Source: CAD feature listing. Evaluate the final solid. Frame: model axes, mm. A direction names the side the tool comes from. Round coordinates to 2 decimals unless told otherwise and drop trailing zeros. Order: outer loops, then holes, each group sorted by start corner. A loop starts at its lowest first (then second) coordinate and runs counter-clockwise, first axis right, second up. Notation, with made-up numbers: M -18,9.25 L 32,9.25 A24 ccw 32,44.25 Z; hole C -13,18 d11. An arc over 180 degrees is marked long. Answer as CSV lines item,"result". Start each with the question number.
Item 1: Line query: line 1 (Z direction, x = 13, y = 28); line 2 (Z direction, x = 4, y = 34); line 3 (Z direction, x = 3.5, y = 13). Output: solid intervals per line, ascending. Write a range as [from, to].
Item 2: Section query B-B on x = 11.6. Return the cut outline in (y, z), plus the area to 3 significant figures.
Item 3: Pull-direction query (X, two-part tool) for faces 5 (the face through (12, 0, 15)), 6 (the face through (11.65, 4.33, -15.21)), 7 (the face through (-12.747, 33.699, -0.28)); classes: +X half, -X half, draft (parallel to the pull), parting line (faces both ways), or undercut.
Item 4: First-contact query: P1, Ø0.6, axis at y = 0.5, z = -14.5, coming from the +X side; P2, Ø3, axis at x = 3, z = -16, coming from the +Y side; P3, Ø1.6, axis at y = 1, z = -14, coming from the -X side. Flat tips, straight axial feed; report the tip coordinate or a pass-through.
Item 5: Section query A-A on y = 26.5. Return the cut outline in (x, z), plus the area to 3 significant figures.
Item 6: Set-up query: faces 1 (the face through (35.947, 33.699, 0.28)), 2 (the face through (12, 38, -2.55)), 3 (the face through (-10.747, 16.146, -0.236)), 4 (the face through (11.8, 45.7, 7.4)). Return all of +Z, -Z, +X, -X, +Y, -Y with unobstructed straight access to the full face (end or side cutting, diameter ignored); none if empty.
from build123d import *

# Parameters (mm, degrees)
BOSS_EXTRUDE1_DEPTH     = 53.5
BOSS_EXTRUDE2_START     = 32.75
BOSS_EXTRUDE2_DEPTH     = 10
BOSS_EXTRUDE3_DEPTH     = 2
FILLET1_R               = 10.75
FILLET2_R               = 14
FILLET3_R               = 1
CUT_EXTRUDE4_DEPTH      = 79.076260797
CUT_EXTRUDE5_DEPTH      = 61.840180017
CUT_EXTRUDE5_DEPTH_BACK = 61.840180017


# Some blends are built 0.0001 mm under size
with BuildPart() as part:
    # Sketch2 → Boss-Extrude1 (new body)
    with BuildSketch(Plane(origin=(0, 0, 0), x_dir=(1, 0, 0), z_dir=(0, 1, 0))):
        with BuildLine():
            Line((0, -12.75), (23.2, -12.75))
            ThreePointArc((23.2, -12.75), (35.95, 0), (23.2, 12.75))
            Line((23.2, 12.75), (0, 12.75))
            ThreePointArc((0, 12.75), (-12.75, 0), (0, -12.75))
        make_face()
        with BuildLine():
            ThreePointArc((23.2, -10.75), (33.95, 0), (23.2, 10.75))
            Line((23.2, 10.75), (0, 10.75))
            ThreePointArc((0, 10.75), (-10.75, 0), (0, -10.75))
            Line((0, -10.75), (23.2, -10.75))
        make_face(mode=Mode.SUBTRACT)
    extrude(amount=BOSS_EXTRUDE1_DEPTH)

    # Sketch2<3> → Boss-Extrude2 (add)
    with BuildSketch(Plane(origin=(0, 0, 0), x_dir=(1, 0, 0), z_dir=(0, 1, 0)).offset(BOSS_EXTRUDE2_START)):
        with BuildLine():
            Line((0, -10.75), (23.2, -10.75))
            ThreePointArc((23.2, -10.75), (33.95, 0), (23.2, 10.75))
            Line((23.2, 10.75), (0, 10.75))
            ThreePointArc((0, 10.75), (-10.75, 0), (0, -10.75))
        make_face()
    extrude(amount=BOSS_EXTRUDE2_DEPTH)

    # Sketch2<4> → Boss-Extrude3 (add)
    with BuildSketch(Plane(origin=(0, 0, 0), x_dir=(1, 0, 0), z_dir=(0, 1, 0))):
        with BuildLine():
            Line((0, 22.75), (23.2, 22.75))
            ThreePointArc((23.2, 22.75), (45.95, 0), (23.2, -22.75))
            Line((23.2, -22.75), (0, -22.75))
            ThreePointArc((0, -22.75), (-22.75, 0), (0, 22.75))
        make_face()
        with BuildLine():
            ThreePointArc((23.2, -12.75), (35.95, 0), (23.2, 12.75))
            Line((23.2, 12.75), (0, 12.75))
            ThreePointArc((0, 12.75), (-12.75, 0), (0, -12.75))
            Line((0, -12.75), (23.2, -12.75))
        make_face(mode=Mode.SUBTRACT)
    extrude(amount=BOSS_EXTRUDE3_DEPTH)

    # Fillet1
    fillet1_edges = [part.edges().sort_by_distance(p)[0] for p in [
        (11.6, 42.75, -10.75),
        (33.95, 42.75, 0),
        (11.6, 42.75, 10.75),
        (-10.75, 42.75, 0),
    ]]
    fillet(fillet1_edges, radius=FILLET1_R - 0.0001)  # a hair under: the kernel refuses the full size

    # Fillet2
    # the kernel refuses this fillet: 14 mm, written as the material it adds along each edge
    with BuildSketch(Plane(origin=(23.2, 2, 0), x_dir=(0, 0, 1), z_dir=(-1, 0, 0))) as fillet2_piece_1:
        with BuildLine():
            CenterArc((26.75, 13.416407865), FILLET2_R, 180, 73.398450401)
            Line((22.75, 0), (22.67, -0.268328157))
            ThreePointArc((22.67, -0.268328157), (17.75, -0.28), (12.75, -0.28))
            Line((12.75, -0.28), (12.47, 0))
            Line((12.47, 0), (12.47, 13.416407865))
            Line((12.47, 13.416407865), (12.75, 13.416407865))
        make_face()
    revolve(axis=Axis((23.2, 2, 0), (0, 1, 0)), revolution_arc=180)
    with BuildSketch(Plane(origin=(0, 2, 12.75), x_dir=(0, 1, 0), z_dir=(1, 0, 0)), Plane(origin=(23.2, 2, -12.75), x_dir=(0, 1, 0), z_dir=(-1, 0, 0))) as fillet2_piece_2:
        with BuildLine():
            CenterArc((13.416407865, 14), FILLET2_R, 196.601549599, 73.398450401)
            Line((0, 10), (-0.268328157, 9.92))
            ThreePointArc((-0.268328157, 9.92), (-0.28, 5), (-0.28, 0))
            Line((-0.28, 0), (0, -0.28))
            Line((0, -0.28), (13.416407865, -0.28))
            Line((13.416407865, -0.28), (13.416407865, 0))
        make_face()
    extrude(amount=23.2)
    with BuildSketch(Plane(origin=(0, 2, 0), x_dir=(0, 0, -1), z_dir=(1, 0, 0))) as fillet2_piece_3:
        with BuildLine():
            CenterArc((26.75, 13.416407865), FILLET2_R, 180, 73.398450401)
            Line((22.75, 0), (22.67, -0.268328157))
            ThreePointArc((22.67, -0.268328157), (17.75, -0.28), (12.75, -0.28))
            Line((12.75, -0.28), (12.47, 0))
            Line((12.47, 0), (12.47, 13.416407865))
            Line((12.47, 13.416407865), (12.75, 13.416407865))
        make_face()
    revolve(axis=Axis((0, 2, 0), (0, 1, 0)), revolution_arc=180)

    # Fillet3
    # the kernel refuses this fillet: 1 mm, written as the material it takes off along each edge
    with BuildSketch(Plane(origin=(0, 53.5, 10.75), x_dir=(0, 0, 1), z_dir=(1, 0, 0)), Plane(origin=(23.2, 53.5, -10.75), x_dir=(0, 0, -1), z_dir=(-1, 0, 0))) as fillet3_piece_1:
        with BuildLine():
            CenterArc((0.957377651, 1), FILLET3_R, 184.881694581, 85.118305419)
            Line((-0.038994884, 0.914901403), (-0.138632138, 0.906391544))
            ThreePointArc((-0.138632138, 0.906391544), (-0.1, 0.0001), (-0.1, 0))
            Line((-0.1, 0), (0, -0.1))
            Line((0, -0.1), (0.957377651, -0.1))
            Line((0.957377651, -0.1), (0.957377651, 0))
        make_face()
    extrude(amount=23.2, mode=Mode.SUBTRACT)
    with BuildSketch(Plane(origin=(0, 53.5, 0), x_dir=(0, 0, -1), z_dir=(1, 0, 0))) as fillet3_piece_2:
        with BuildLine():
            CenterArc((11.707377651, -1), FILLET3_R, 90, 85.118305419)
            Line((10.711005116, -0.914901403), (10.611367862, -0.906391544))
            ThreePointArc((10.611367862, -0.906391544), (10.65, -0.0001), (10.65, 0))
            Line((10.65, 0), (10.75, 0.1))
            Line((10.75, 0.1), (11.707377651, 0.1))
            Line((11.707377651, 0.1), (11.707377651, 0))
        make_face()
    revolve(axis=Axis((0, 53.5, 0), (0, 1, 0)), revolution_arc=180, mode=Mode.SUBTRACT)
    with BuildSketch(Plane(origin=(0, 53.5, 12.75), x_dir=(0, -1, 0), z_dir=(1, 0, 0))) as fillet3_piece_3:
        with BuildLine():
            CenterArc((FILLET3_R, FILLET3_R), FILLET3_R, 180, 90)
            Line((0, FILLET3_R), (0, 0))
            Line((0, 0), (FILLET3_R, 0))
        make_face()
    extrude(amount=23.2, mode=Mode.SUBTRACT)
    with BuildSketch(Plane(origin=(23.2, 53.5, 0), x_dir=(0, 0, 1), z_dir=(-1, 0, 0))) as fillet3_piece_4:
        with BuildLine():
            CenterArc((12.75 - FILLET3_R, -FILLET3_R), FILLET3_R, 0, 90)
            Line((12.75, -FILLET3_R), (12.75, 0))
            Line((12.75, 0), (12.75 - FILLET3_R, 0))
        make_face()
    revolve(axis=Axis((23.2, 53.5, 0), (0, 1, 0)), revolution_arc=180, mode=Mode.SUBTRACT)
    with BuildSketch(Plane(origin=(23.2, 53.5, -12.75), x_dir=(0, 0, 1), z_dir=(-1, 0, 0))) as fillet3_piece_5:
        with BuildLine():
            CenterArc((FILLET3_R, -FILLET3_R), FILLET3_R, 90, 90)
            Line((0, -FILLET3_R), (0, 0))
            Line((0, 0), (FILLET3_R, 0))
        make_face()
    extrude(amount=23.2, mode=Mode.SUBTRACT)
    with BuildSketch(Plane(origin=(0, 53.5, 0), x_dir=(0, 0, -1), z_dir=(1, 0, 0))) as fillet3_piece_6:
        with BuildLine():
            CenterArc((12.75 - FILLET3_R, -FILLET3_R), FILLET3_R, 0, 90)
            Line((12.75 - FILLET3_R, 0), (12.75, 0))
            Line((12.75, 0), (12.75, -FILLET3_R))
        make_face()
    revolve(axis=Axis((0, 53.5, 0), (0, 1, 0)), revolution_arc=180, mode=Mode.SUBTRACT)
    with BuildSketch(Plane(origin=(0, 2, -22.75), x_dir=(0, 0.30962089103713925, 0.9508600863604318), z_dir=(1, 0, 0)), Plane(origin=(23.2, 2, 22.75), x_dir=(0, 0.30962089103713925, -0.9508600863604318), z_dir=(-1, 0, 0))) as fillet3_piece_7:
        with BuildLine():
            CenterArc((0.726159611, 0.99968645), FILLET3_R, 198.036385117, 70.528779366)
            Line((-0.224700475, 0.690065559), (0, 0))
            ThreePointArc((0, 0), (0.350559812, 0.004389695), (0.701119624, 0))
        make_face()
    extrude(amount=23.2, mode=Mode.SUBTRACT)
    with BuildSketch(Plane(origin=(0, 2, 0), x_dir=(0, 0, 1), z_dir=(1, 0, 0))) as fillet3_piece_8:
        with BuildLine():
            CenterArc((21.75, 0.725727759), FILLET3_R, 289.471220634, 70.528779366)
            Line((22.75, 0.725727759), (22.75, 0))
            ThreePointArc((22.75, 0), (22.415307525, -0.104366656), (22.083333333, -0.217081283))
        make_face()
    revolve(axis=Axis((0, 2, 0), (0, -1, 0)), revolution_arc=180, mode=Mode.SUBTRACT)
    with BuildSketch(Plane(origin=(23.2, 2, 0), x_dir=(0, 0, -1), z_dir=(-1, 0, 0))) as fillet3_piece_9:
        with BuildLine():
            CenterArc((21.75, 0.725727759), FILLET3_R, 289.471220634, 70.528779366)
            Line((22.75, 0.725727759), (22.75, 0))
            ThreePointArc((22.75, 0), (22.415307525, -0.104366656), (22.083333333, -0.217081283))
        make_face()
    revolve(axis=Axis((23.2, 2, 0), (0, -1, 0)), revolution_arc=180, mode=Mode.SUBTRACT)
    with BuildSketch(Plane(origin=(23.2, 53.5, 0), x_dir=(0, 0, 1), z_dir=(-1, 0, 0))) as fillet3_piece_10:
        with BuildLine():
            CenterArc((11.707377651, -1), FILLET3_R, 90, 85.118305419)
            Line((10.711005116, -0.914901403), (10.611367862, -0.906391544))
            ThreePointArc((10.611367862, -0.906391544), (10.65, -0.0001), (10.65, 0))
            Line((10.65, 0), (10.75, 0.1))
            Line((10.75, 0.1), (11.707377651, 0.1))
            Line((11.707377651, 0.1), (11.707377651, 0))
        make_face()
    revolve(axis=Axis((23.2, 53.5, 0), (0, 1, 0)), revolution_arc=180, mode=Mode.SUBTRACT)

    # Sketch4 → Cut-Extrude4 (cut, through all)
    with BuildSketch(Plane.XY.offset(-10.75)):
        with BuildLine():
            Line((11.6, 0), (12.85, 0))
            Line((12.85, 0), (12.85, 2.002168665))
            ThreePointArc((12.85, 2.002168665), (11.6, 4.331324862), (10.35, 2.002168665))
            Line((10.35, 2.002168665), (10.35, 0))
            Line((10.35, 0), (11.6, 0))
        make_face()
    extrude(amount=-CUT_EXTRUDE4_DEPTH, mode=Mode.SUBTRACT)

    # Sketch3 → Cut-Extrude5 (cut, two sides: drawn at the far end of the back side and taken through both)
    with BuildSketch(Plane.XZ.offset(-32.75).offset(-CUT_EXTRUDE5_DEPTH_BACK)):
        with BuildLine():
            Line((12.95, 2.55), (10.25, 2.55))
            ThreePointArc((10.25, 2.55), (7.7, 0), (10.25, -2.55))
            Line((10.25, -2.55), (12.95, -2.55))
            ThreePointArc((12.95, -2.55), (15.5, 0), (12.95, 2.55))
        make_face()
    extrude(amount=CUT_EXTRUDE5_DEPTH + CUT_EXTRUDE5_DEPTH_BACK, mode=Mode.SUBTRACT)


solid = part.part
Results:
1,line 1,"[-12.75, -10.75], [10.75, 12.75]"
1,line 2,"[-12.75, 12.75]"
1,line 3,"[-12.96, -10.75], [10.75, 12.96]"
2,outline,"M 0,10.75 L 32.75,10.75 L 32.75,2.55 L 43.06,2.55 A10.75 cw 52.59,10.71 A1 ccw 53.5,11.71 L 53.5,11.75 A1 ccw 52.5,12.75 L 15.42,12.75 A14 cw 2.22,22.08 A1 ccw 1.27,22.75 L 0,22.75 Z; M 4.33,-18.2 A14 cw 15.42,-12.75 L 52.5,-12.75 A1 ccw 53.5,-11.75 L 53.5,-11.71 A1 ccw 52.59,-10.71 A10.75 cw 43.06,-2.55 L 32.75,-2.55 L 32.75,-10.75 L 4.33,-10.75 Z"
2,area,"491 mm^2"
3,face 5,"draft"
3,face 6,"undercut"
3,face 7,"-X half"
4,P1,"x = 40.97"
4,P2,"y = 8.64"
4,P3,"x = -18.53"
5,outline,"M 0,-12.75 L 23.2,-12.75 A12.75 ccw 23.2,12.75 L 0,12.75 A12.75 ccw Z; hole M 0,-10.75 L 23.2,-10.75 A10.75 ccw 23.2,10.75 L 0,10.75 A10.75 ccw Z"
5,area,"240 mm^2"
6,face 1,"+X, +Y"
6,face 2,"+Y, -Y"
6,face 3,"-Y"
6,face 4,"+Y"
